```python
from build123d import *

# Parameters (mm, degrees)
SKETCH1_R                      = 3.5
BOSS_EXTRUDE1_DEPTH            = 21
SKETCH4_R                      = 25
BOSS_EXTRUDE2_DEPTH            = 18
CUT_EXTRUDE2_DEPTH             = 20
SKETCH7_R                      = 2.125
CUT_EXTRUDE3_DEPTH             = 105.070425208
SKETCH9_R                      = 4
CUT_EXTRUDE4_DEPTH             = 36
CUT_EXTRUDE4_DIRECTION_2_REACH = 91.556
SKETCH10_R                     = 2.125
BOSS_EXTRUDE3_DEPTH            = 10


with BuildPart() as part:
    # Sketch1 → Boss-Extrude1 (new body)
    with BuildSketch(Plane.XY):
        with BuildLine():
            ThreePointArc((-27.16441994, 47.550254291), (-29.67571676, 44.192804958), (-33.605829095, 45.653385243))
            Line((-33.605829095, 45.653385243), (-25.93972411, 33.765821671))
            ThreePointArc((-25.93972411, 33.765821671), (-24.90753088, 12.791204222), (-42.555985811, 1.409989939))
            Line((-42.555985811, 1.409989939), (-56.683970347, 0.71473006))
            ThreePointArc((-56.683970347, 0.71473006), (-54.098653318, -0.246072778), (-53.011938142, -2.781039515))
            ThreePointArc((-53.011938142, -2.781039515), (-53.976971405, -5.194324339), (-56.339905937, -6.27680909))
            Line((-56.339905937, -6.27680909), (-42.211921401, -5.581549211))
            ThreePointArc((-42.211921401, -5.581549211), (-23.531273241, -15.174952377), (-22.499080012, -36.149569826))
            Line((-22.499080012, -36.149569826), (-28.960959562, -48.732393278))
            ThreePointArc((-28.960959562, -48.732393278), (-25.025035607, -46.929305801), (-22.347518202, -50.331293805))
            ThreePointArc((-22.347518202, -50.331293805), (-22.445530198, -51.153776401), (-22.734076842, -51.930194333))
            Line((-22.734076842, -51.930194333), (-16.272197292, -39.347370882))
            ThreePointArc((-16.272197292, -39.347370882), (1.376257639, -27.966156599), (20.0569058, -37.559559765))
            Line((20.0569058, -37.559559765), (27.723010785, -49.447123338))
            ThreePointArc((27.723010785, -49.447123338), (28.767550893, -44.608845135), (33.605829095, -45.653385243))
            Line((33.605829095, -45.653385243), (25.93972411, -33.765821671))
            ThreePointArc((25.93972411, -33.765821671), (24.90753088, -12.791204222), (42.555985811, -1.409989939))
            Line((42.555985811, -1.409989939), (56.683970347, -0.71473006))
            ThreePointArc((56.683970347, -0.71473006), (53.016168567, 2.60900731), (56.339905937, 6.27680909))
            Line((56.339905937, 6.27680909), (42.211921401, 5.581549211))
            ThreePointArc((42.211921401, 5.581549211), (23.531273241, 15.174952377), (22.499080012, 36.149569826))
            Line((22.499080012, 36.149569826), (28.960959562, 48.732393278))
            ThreePointArc((28.960959562, 48.732393278), (24.248617674, 47.217852445), (22.734076842, 51.930194333))
            Line((22.734076842, 51.930194333), (16.272197292, 39.347370882))
            ThreePointArc((16.272197292, 39.347370882), (-1.376257639, 27.966156599), (-20.0569058, 37.559559765))
            Line((-20.0569058, 37.559559765), (-27.723010785, 49.447123338))
            ThreePointArc((-27.723010785, 49.447123338), (-27.306970607, 48.538957471), (-27.16441994, 47.550254291))
        make_face()
        with Locations((-56.511938142, -2.781039515)):
            Circle(SKETCH1_R)
        with Locations((-30.66441994, 47.550254291)):
            Circle(SKETCH1_R)
        with Locations((25.847518202, 50.331293805)):
            Circle(SKETCH1_R)
        with Locations((56.511938142, 2.781039515)):
            Circle(SKETCH1_R)
        with Locations((30.66441994, -47.550254291)):
            Circle(SKETCH1_R)
        with Locations((-25.847518202, -50.331293805)):
            Circle(SKETCH1_R)
    extrude(amount=BOSS_EXTRUDE1_DEPTH)

    # Sketch3 → Revolve1 (revolve)
    with BuildSketch(Plane(origin=(0, 0, 0), x_dir=(-0.9987913071010414, -0.04915205854685543, 0), z_dir=(0.04915205854685543, -0.9987913071010414, 0)), mode=Mode.PRIVATE) as revolve1_sk:
        Polygon((0, 0), (-28, 0), (0, 26.813467396), align=None)
    revolve(revolve1_sk.sketch.rotate(Axis((0, 0, -26.813467396), (0, 0, 1)), 357.182659299), axis=Axis((0, 0, -26.813467396), (0, 0, 1)))

    # Sketch4 → Boss-Extrude2 (add)
    with BuildSketch(Plane.XY.offset(21)):
        Circle(SKETCH4_R)
    extrude(amount=BOSS_EXTRUDE2_DEPTH)

    # Sketch5 → Cut-Extrude2 (cut)
    with BuildSketch(Plane.XY.offset(39)):
        with BuildLine():
            Line((-1.658312395, 2.5), (1.658312395, 2.5))
            ThreePointArc((1.658312395, 2.5), (0, -3), (-1.658312395, 2.5))
        make_face()
    extrude(amount=-CUT_EXTRUDE2_DEPTH, mode=Mode.SUBTRACT)

    # Sketch7 → Cut-Extrude3 (cut, through all)
    with BuildSketch(Plane.XY.offset(39)):
        with Locations((-8, 8)):
            Circle(SKETCH7_R)
        with Locations(Location((8, 8, 0), (0, 0, 225))):
            Circle(SKETCH7_R)
        with Locations((8, -8)):
            Circle(SKETCH7_R)
        with Locations(Location((-8, -8, 0), (0, 0, 110.081495148))):
            Circle(SKETCH7_R)
    extrude(amount=-CUT_EXTRUDE3_DEPTH, mode=Mode.SUBTRACT)

    # Sketch9 → Cut-Extrude4 (cut)
    with BuildSketch(Plane(origin=(0, 0, 0), x_dir=(-1, 0, 0), z_dir=(0, 0, -1))):
        with Locations(Location((-8, 8, 0), (0, 0, 315))):
            Circle(SKETCH9_R)
        with Locations(Location((8, 8, 0), (0, 0, 225))):
            Circle(SKETCH9_R)
        with Locations(Location((8, -8, 0), (0, 0, 135))):
            Circle(SKETCH9_R)
        with Locations(Location((-8, -8, 0), (0, 0, 45))):
            Circle(SKETCH9_R)
    extrude(amount=-CUT_EXTRUDE4_DEPTH, mode=Mode.SUBTRACT)

    # Cut-Extrude4 direction 2: up to this cone (the profile starts inside it)
    cut_extrude4_direction_2_end = Plane(origin=(0, 0, 0), z_dir=(0, 0, 1)).offset(-26.813466396) * Cone(1.044e-06, 153.368642194, 146.869466396, align=(Align.CENTER, Align.CENTER, Align.MIN), mode=Mode.PRIVATE)
    # Sketch9 → Cut-Extrude4 direction 2 (cut, up to the surface)
    with BuildSketch(Plane(origin=(0, 0, 0), x_dir=(-1, 0, 0), z_dir=(0, 0, -1)), mode=Mode.PRIVATE) as cut_extrude4_direction_2_sk1:
        with Locations(Location((-8, 8, 0), (0, 0, 315))):
            Circle(SKETCH9_R)
    cut_extrude4_direction_2_tool1 = extrude(cut_extrude4_direction_2_sk1.sketch, amount=CUT_EXTRUDE4_DIRECTION_2_REACH, mode=Mode.PRIVATE) & cut_extrude4_direction_2_end
    add(cut_extrude4_direction_2_tool1.solids().sort_by_distance((8, 8, 0))[0], mode=Mode.SUBTRACT)
    # Sketch9 → Cut-Extrude4 direction 2 (cut, up to the surface)
    with BuildSketch(Plane(origin=(0, 0, 0), x_dir=(-1, 0, 0), z_dir=(0, 0, -1)), mode=Mode.PRIVATE) as cut_extrude4_direction_2_sk2:
        with Locations(Location((8, 8, 0), (0, 0, 225))):
            Circle(SKETCH9_R)
    cut_extrude4_direction_2_tool2 = extrude(cut_extrude4_direction_2_sk2.sketch, amount=CUT_EXTRUDE4_DIRECTION_2_REACH, mode=Mode.PRIVATE) & cut_extrude4_direction_2_end
    add(cut_extrude4_direction_2_tool2.solids().sort_by_distance((-8, 8, 0))[0], mode=Mode.SUBTRACT)
    # Sketch9 → Cut-Extrude4 direction 2 (cut, up to the surface)
    with BuildSketch(Plane(origin=(0, 0, 0), x_dir=(-1, 0, 0), z_dir=(0, 0, -1)), mode=Mode.PRIVATE) as cut_extrude4_direction_2_sk3:
        with Locations(Location((8, -8, 0), (0, 0, 135))):
            Circle(SKETCH9_R)
    cut_extrude4_direction_2_tool3 = extrude(cut_extrude4_direction_2_sk3.sketch, amount=CUT_EXTRUDE4_DIRECTION_2_REACH, mode=Mode.PRIVATE) & cut_extrude4_direction_2_end
    add(cut_extrude4_direction_2_tool3.solids().sort_by_distance((-8, -8, 0))[0], mode=Mode.SUBTRACT)
    # Sketch9 → Cut-Extrude4 direction 2 (cut, up to the surface)
    with BuildSketch(Plane(origin=(0, 0, 0), x_dir=(-1, 0, 0), z_dir=(0, 0, -1)), mode=Mode.PRIVATE) as cut_extrude4_direction_2_sk4:
        with Locations(Location((-8, -8, 0), (0, 0, 45))):
            Circle(SKETCH9_R)
    cut_extrude4_direction_2_tool4 = extrude(cut_extrude4_direction_2_sk4.sketch, amount=CUT_EXTRUDE4_DIRECTION_2_REACH, mode=Mode.PRIVATE) & cut_extrude4_direction_2_end
    add(cut_extrude4_direction_2_tool4.solids().sort_by_distance((8, -8, 0))[0], mode=Mode.SUBTRACT)

    # Sketch10 → Boss-Extrude3 (add)
    with BuildSketch(Plane.XY.offset(21)):
        with BuildLine():
            Line((-22.499080012, -36.149569826), (-28.960959562, -48.732393278))
            ThreePointArc((-28.960959562, -48.732393278), (-27.44641873, -53.444735165), (-22.734076842, -51.930194333))
            Line((-22.734076842, -51.930194333), (-16.272197292, -39.347370882))
            ThreePointArc((-16.272197292, -39.347370882), (1.376257639, -27.966156599), (20.0569058, -37.559559765))
            Line((20.0569058, -37.559559765), (27.723010785, -49.447123338))
            ThreePointArc((27.723010785, -49.447123338), (32.561288987, -50.491663446), (33.605829095, -45.653385243))
            Line((33.605829095, -45.653385243), (25.93972411, -33.765821671))
            ThreePointArc((25.93972411, -33.765821671), (24.90753088, -12.791204222), (42.555985811, -1.409989939))
            Line((42.555985811, -1.409989939), (56.683970347, -0.71473006))
            ThreePointArc((56.683970347, -0.71473006), (60.007707717, 2.95307172), (56.339905937, 6.27680909))
            Line((56.339905937, 6.27680909), (42.211921401, 5.581549211))
            ThreePointArc((42.211921401, 5.581549211), (23.531273241, 15.174952377), (22.499080012, 36.149569826))
            Line((22.499080012, 36.149569826), (28.960959562, 48.732393278))
            ThreePointArc((28.960959562, 48.732393278), (27.44641873, 53.444735165), (22.734076842, 51.930194333))
            Line((22.734076842, 51.930194333), (16.272197292, 39.347370882))
            ThreePointArc((16.272197292, 39.347370882), (-1.376257639, 27.966156599), (-20.0569058, 37.559559765))
            Line((-20.0569058, 37.559559765), (-27.723010785, 49.447123338))
            ThreePointArc((-27.723010785, 49.447123338), (-32.561288987, 50.491663446), (-33.605829095, 45.653385243))
            Line((-33.605829095, 45.653385243), (-25.93972411, 33.765821671))
            ThreePointArc((-25.93972411, 33.765821671), (-24.90753088, 12.791204222), (-42.555985811, 1.409989939))
            Line((-42.555985811, 1.409989939), (-56.683970347, 0.71473006))
            ThreePointArc((-56.683970347, 0.71473006), (-60.007707717, -2.95307172), (-56.339905937, -6.27680909))
            Line((-56.339905937, -6.27680909), (-42.211921401, -5.581549211))
            ThreePointArc((-42.211921401, -5.581549211), (-23.531273241, -15.174952377), (-22.499080012, -36.149569826))
        make_face()
        with Locations((8, -8)):
            Circle(SKETCH10_R, mode=Mode.SUBTRACT)
        with Locations((-8, -8)):
            Circle(SKETCH10_R, mode=Mode.SUBTRACT)
        with Locations((8, 8)):
            Circle(SKETCH10_R, mode=Mode.SUBTRACT)
        with Locations((-8, 8)):
            Circle(SKETCH10_R, mode=Mode.SUBTRACT)
        with BuildLine():
            Line((-1.658312395, 2.5), (1.658312395, 2.5))
            ThreePointArc((1.658312395, 2.5), (0, -3), (-1.658312395, 2.5))
        make_face(mode=Mode.SUBTRACT)
    extrude(amount=BOSS_EXTRUDE3_DEPTH)


solid = part.part
```
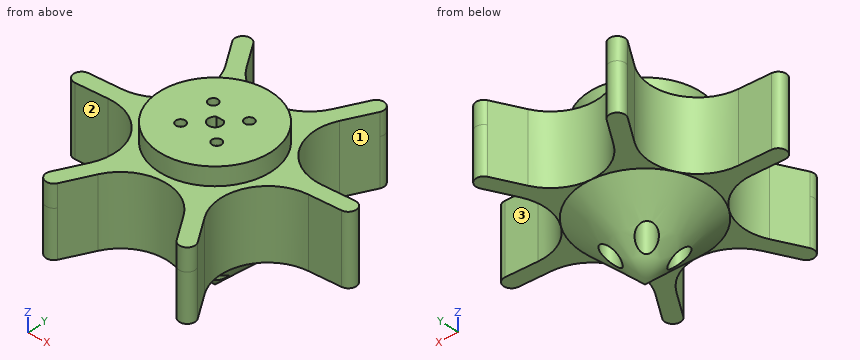
Geometry check sheet. Reference: the model listing, model coordinates, mm. Face numbers are marked on the shaded views. A direction names the side the tool comes from. Coordinates: 2 decimals unless noted, no trailing zeros. Loops run counter-clockwise (first coordinate to the right, second up) from the corner with the lowest first, then second, coordinate; pieces in that order, holes last.
Item 1: Access from +Z, -Z, +X, -X, +Y, -Y to the whole of each face (thin tool, end or side, straight path). Record for the marked faces 1, 2 and 3.
Item 2: Thickness scan on line 1 (Y direction, x = 8, z = -6); line 2 (Y direction, x = 8, z = 32.25); line 3 (X direction, y = -9, z = 7). Record the ranges inside material, lowest first.
Item 3: Sectioned sample at A-A, the plane z = 33.5. Record the boundary of the cut face in (x, y), then the cut area to 3 significant figures.
Item 4: Sectioned sample at C-C, the plane y = 8. Count the separate pieces of the cut face and the enclosed holes in it, then the cut area to 3 significant figures.
Item 5: Sectioned sample at D-D, the plane z = -17.5. Record the boundary of the cut face in (x, y), then the cut area to 3 significant figures.
Item 6: Sectioned sample at B-B, the plane z = 5.5. Record the boundary of the cut face in (x, y).
Item 7: Go/stop test with flat-tipped pins: pin 1 Ø6 at (x, z) = (42, 27.5) entering from +Y; pin 2 Ø4 at (x, y) = (20, 19.5) entering from +Z; pin 3 Ø4 at (x, z) = (-44, 25.5) entering from -Y; pin 4 Ø13 at (x, y) = (8, 8) entering from +Z. Record where each tip stops, or that it passes through.
Check result:
1. face 1: +Z, -Z, +X
1. face 2: +Z, -Z, -Y
1. face 3: +Z, -Z, +Y
2. line 1: y = -20.21 to -12, -4 to 4, 12 to 20.21
2. line 2: y = -23.69 to -12, -4 to 4, 12 to 23.69
2. line 3: x = -29.66 to -11.87, -4.13 to 4.13, 11.87 to 27.41
3. outline: circle Ø50 at (0, 0); hole circle Ø8 at (-8, -8); hole circle Ø8 at (-8, 8); hole (-1.66, 2.5) arc R3 ccw (long way) to (1.66, 2.5) - close; hole circle Ø8 at (8, -8); hole circle Ø8 at (8, 8)
3. area: 1,740 mm2
4. separate pieces: 3
4. enclosed holes: 0
4. area: 2,050 mm2
5. outline: (-8.83, -4.09) arc R4 cw to (-4.09, -8.83) arc R9.73 ccw to (4.09, -8.83) arc R4 cw to (8.83, -4.09) arc R9.73 ccw to (8.83, 4.09) arc R4 cw to (4.09, 8.83) arc R9.73 ccw to (-4.09, 8.83) arc R4 cw to (-8.83, 4.09) arc R9.73 ccw to start
5. area: 252 mm2
6. outline: (-56.68, 0.71) arc R3.5 ccw to (-56.34, -6.28) - (-42.21, -5.58) arc R21 cw to (-22.5, -36.15) - (-28.96, -48.73) arc R3.5 ccw to (-22.73, -51.93) - (-16.27, -39.35) arc R21 cw to (20.06, -37.56) - (27.72, -49.45) arc R3.5 ccw to (33.61, -45.65) - (25.94, -33.77) arc R21 cw to (42.56, -1.41) - (56.68, -0.71) arc R3.5 ccw to (56.34, 6.28) - (42.21, 5.58) arc R21 cw to (22.5, 36.15) - (28.96, 48.73) arc R3.5 ccw to (22.73, 51.93) - (16.27, 39.35) arc R21 cw to (-20.06, 37.56) - (-27.72, 49.45) arc R3.5 ccw to (-33.61, 45.65) - (-25.94, 33.77) arc R21 cw to (-42.56, 1.41) - close; hole circle Ø8 at (-8, -8); hole circle Ø8 at (-8, 8); hole circle Ø8 at (8, -8); hole circle Ø8 at (8, 8)
7. pin 1: stops at y = 5.72
7. pin 2: stops at z = 31
7. pin 3: stops at y = -5.77
7. pin 4: stops at z = 39
